Can you work these out from the drawing? Everything is in mm from the part's minimum corner. A direction names the side the tool comes from. Round coordinates to 2 decimals unless told otherwise and drop trailing zeros. Write each loop counter-clockwise with the first axis right and the second up, starting at its lowest first coordinate (ties: lowest second). Pieces come first, ordered by that corner, then holes.
Q1. For the marked faces 1 and 2, which set-ups out of +Z, -Z, +X, -X, +Y, -Y let a thin tool reach every point of the face, with its end or its side?
Q2. If we section it at B-B (x = 12): Please give me the cut outline in (y, z).
Q3. I'm going to push flat-ended pins straight in: pin 1 Ø2 at (y, z) = (15.5, 5.5) entering from +X; pin 2 Ø4 at (x, z) = (11, 2.5) entering from +Y; pin 3 Ø8 at (x, y) = (19.5, 75.5) entering from +Z; pin 4 Ø12 at (x, z) = (11.5, 7.5) entering from +Y. Where does each tip first touch, or does it pass through?
Q4. If we section it at D-D (y = 39): Please give me the cut outline in (x, z).
Q5. Please list where these lines run through material, in increasing order: line 1 along Y through (x, z) = (19, 4); line 2 along Z through (x, y) = (9.5, 29); line 3 along X through (y, z) = (9.5, 11).
Q6. If we section it at A-A (z = 18): Please give me the cut outline in (x, y).
Q7. If we section it at C-C (z = 12): Please give me the cut outline in (x, y), plus the area to 3 significant figures.
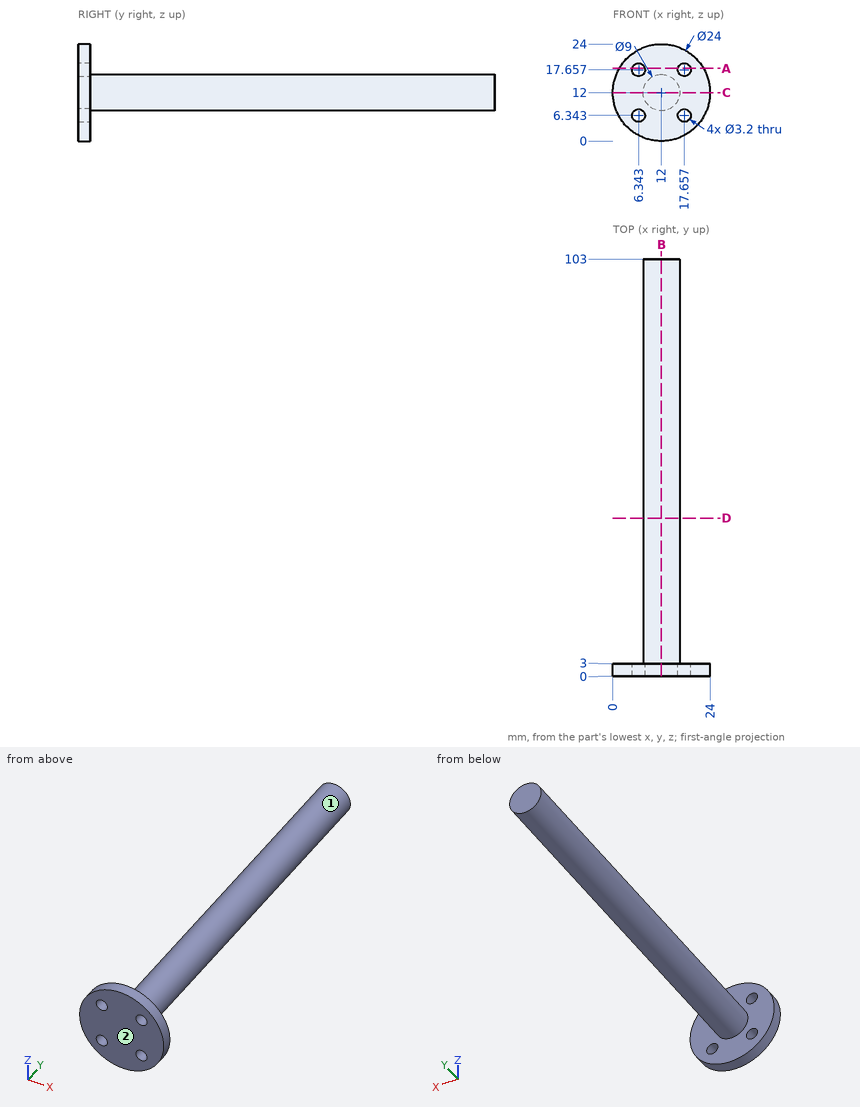
A:
1. face 1: +Y
1. face 2: +Z, -Z, +X, -X, -Y
2. outline: (0, 0) - (3, 0) - (3, 7.5) - (103, 7.5) - (103, 16.5) - (3, 16.5) - (3, 24) - (0, 24) - close
3. pin 1: passes through
3. pin 2: stops at y = 3
3. pin 3: stops at z = 14.83
3. pin 4: stops at y = 103
4. outline: circle Ø9 at (12, 12)
5. line 1: y = 0 to 3
5. line 2: z = 8.26 to 15.74
5. line 3: x = 7.61 to 16.39
6. outline: (1.61, 0) - (4.78, 0) - (4.78, 3) - (1.61, 3) - close; (7.91, 0) - (16.09, 0) - (16.09, 3) - (7.91, 3) - close; (19.22, 0) - (22.39, 0) - (22.39, 3) - (19.22, 3) - close
7. outline: (0, 0) - (24, 0) - (24, 3) - (16.5, 3) - (16.5, 103) - (7.5, 103) - (7.5, 3) - (0, 3) - close
7. area: 972 mm2
